```python
from build123d import *

# Parameters (mm, degrees)
SKETCH1_R           = 2
BOSS_EXTRUDE1_DEPTH = 2
BOSS_EXTRUDE2_START = -6
SKETCH2_R           = 3.5
SKETCH2_R_2         = 2
BOSS_EXTRUDE2_DEPTH = 4
BOSS_EXTRUDE3_START = 11
BOSS_EXTRUDE3_DEPTH = 11
BOSS_EXTRUDE4_START = -16
SKETCH5_R           = 2
BOSS_EXTRUDE4_DEPTH = 16


with BuildPart() as part:
    # Sketch1 → Boss-Extrude1 (new body)
    with BuildSketch(Plane.XY):
        with BuildLine():
            Line((-17.5, -10), (17.5, -10))
            ThreePointArc((17.5, -10), (23.235764364, -8.191520443), (26.896926208, -3.420201433))
            Line((26.896926208, -3.420201433), (40.065448474, 32.76001614))
            Line((40.065448474, 32.76001614), (-40.065448474, 32.76001614))
            Line((-40.065448474, 32.76001614), (-26.896926208, -3.420201433))
            ThreePointArc((-26.896926208, -3.420201433), (-23.235764364, -8.191520443), (-17.5, -10))
        make_face()
        with Locations((17.5, 0)):
            Circle(SKETCH1_R, mode=Mode.SUBTRACT)
        with Locations((-17.5, 0)):
            Circle(SKETCH1_R, mode=Mode.SUBTRACT)
        with BuildLine():
            Line((2.863480555, 21.190949642), (2.863480555, 7.014373782))
            ThreePointArc((2.863480555, 7.014373782), (0, 4.150893227), (-2.863480555, 7.014373782))
            Line((-2.863480555, 7.014373782), (-2.863480555, 21.190949642))
            ThreePointArc((-2.863480555, 21.190949642), (0, 24.054430197), (2.863480555, 21.190949642))
        make_face(mode=Mode.SUBTRACT)
    extrude(amount=BOSS_EXTRUDE1_DEPTH)

    # Sketch2 → Boss-Extrude2 (add)
    # profile 1 of 2: a face of its own
    with BuildSketch(Plane.XY.offset(2).offset(BOSS_EXTRUDE2_START)):
        with Locations((-17.5, 0)):
            Circle(SKETCH2_R)
        with Locations((-17.5, 0)):
            Circle(SKETCH2_R_2, mode=Mode.SUBTRACT)
    # profile 2 of 2: a face of its own
    with BuildSketch(Plane.XY.offset(2).offset(BOSS_EXTRUDE2_START)):
        with Locations((17.5, 0)):
            Circle(SKETCH2_R)
        with Locations((17.5, 0)):
            Circle(SKETCH2_R_2, mode=Mode.SUBTRACT)
    extrude(amount=BOSS_EXTRUDE2_DEPTH)

    # Sketch4 → Boss-Extrude3 (add)
    with BuildSketch(Plane(origin=(0, 0, 0), x_dir=(-1, 0, 0), z_dir=(0, 0, -1)).offset(BOSS_EXTRUDE3_START)):
        with BuildLine():
            Line((-26.896926208, -3.420201433), (-32.095820312, 10.863642724))
            Line((-32.095820312, 10.863642724), (-30.21643507, 11.547683011))
            Line((-30.21643507, 11.547683011), (-25.017540966, -2.736161147))
            ThreePointArc((-25.017540966, -2.736161147), (-22.088611491, -6.553216354), (-17.5, -8))
            Line((-17.5, -8), (-17.5, -10))
            ThreePointArc((-17.5, -10), (-23.235764364, -8.191520443), (-26.896926208, -3.420201433))
        make_face()
        with BuildLine():
            Line((32.095820312, 10.863642724), (26.896926208, -3.420201433))
            ThreePointArc((26.896926208, -3.420201433), (23.235764364, -8.191520443), (17.5, -10))
            Line((17.5, -10), (17.5, -8))
            ThreePointArc((17.5, -8), (22.088611491, -6.553216354), (25.017540966, -2.736161147))
            Line((25.017540966, -2.736161147), (30.21643507, 11.547683011))
            Line((30.21643507, 11.547683011), (32.095820312, 10.863642724))
        make_face()
    extrude(amount=-BOSS_EXTRUDE3_DEPTH)

    # Sketch5 → Boss-Extrude4 (add)
    with BuildSketch(Plane.XY.offset(2).offset(BOSS_EXTRUDE4_START)):
        with Locations((-17.5, 0)):
            Circle(SKETCH5_R)
        with Locations((17.5, 0)):
            Circle(SKETCH5_R)
    extrude(amount=BOSS_EXTRUDE4_DEPTH)


solid = part.part
```
The model under review builds one solid part; all positions refer to its coordinate system, in mm. A direction names the side the tool comes from. Round coordinates to 2 decimals unless told otherwise and drop trailing zeros. Order: outer loops, then holes, each group sorted by start corner. A loop starts at its lowest first (then second) coordinate and runs counter-clockwise, first axis right, second up. Notation, with made-up numbers: (-37.5, 13.25) -> (-28.5, 13.25) arc R12 cw to (-28.5, 34.25) -> close; hole circle Ø8 at (37, 45.25). An arc over 180 degrees is marked (long way). One line per item, written item: value. Start each with the question number.
Q1. Clearance check with flat-ended pins moving along their axes: pin 1 Ø0.6 at (y, z) = (-9.5, -7.5) entering from +X; pin 2 Ø7.5 at (x, y) = (26.5, 3.5) entering from -Z; pin 3 Ø8 at (x, z) = (-18.5, -6.5) entering from +Y; pin 4 Ø2 at (x, z) = (-11, -0.5) entering from +Y. State where each tip first meets the part, or that it passes through.
Q2. Wall thickness on line 1 (X direction, y = -0.5, z = -5.25); line 2 (Z direction, x = -27.5, y = 15); line 3 (X direction, y = 10, z = -7.25): over which ranges is each line inside the solid? List them lowest first.
Q3. Mouldability with a two-part tool opening along X and no side actions: class faces 5 (the face through (26, -1, -11)), 6 (the face through (20.84, 1.05, -2.03)), 7 (the face through (-23.31, -8.14, -4.59)) as released by +X, released by -X, zero draft, split by the parting line, or undercut.
Q4. Take a section at B-B (x = 0). Write out the cut boundary in (y, z).
Q5. Machinability: for faces 1 (the face through (-31.14, 11.21, -5.58)), 2 (the face through (31.17, 11.2, -5.58)), 3 (the face through (27.653, 4.506, -5.577)), 4 (the face through (-22.032, -6.592, -5.577)), which of the approach directions +Z, -Z, +X, -X, +Y, -Y give a long, thin tool a straight path to every point of the face, cutting with its end or side? Answer none if there is none.
Q6. Take a section at D-D (z = -13). Write out the cut boundary in (x, y).
Q7. Take a section at C-C (y = 13). Write out the cut boundary in (x, z), and give its area (3 significant figures).
Q8. Take a section at A-A (z = -5.75). Write out the cut boundary in (x, y).
Reported:
1. pin 1: stops at x = 21.42
1. pin 2: stops at z = -11
1. pin 3: stops at y = 3.5
1. pin 4: stops at y = 32.76
2. line 1: x = -27.96 to -25.83, -19.44 to -15.56, 15.56 to 19.44, 25.83 to 27.96
2. line 2: z = 0 to 2
2. line 3: x = -31.78 to -29.65, 29.65 to 31.78
3. face 5: zero draft
3. face 6: undercut
3. face 7: released by -X
4. outline: (-10, 0) -> (4.15, 0) -> (4.15, 2) -> (-10, 2) -> close; (24.05, 0) -> (32.76, 0) -> (32.76, 2) -> (24.05, 2) -> close
5. face 1: -Z, -X, +Y
5. face 2: -Z, +X, +Y
5. face 3: -Z, +Y
5. face 4: -Z
6. outline: circle Ø4 at (-17.5, 0); circle Ø4 at (17.5, 0)
7. outline: (-32.87, 0) -> (-2.86, 0) -> (-2.86, 2) -> (-32.87, 2) -> close; (2.86, 0) -> (32.87, 0) -> (32.87, 2) -> (2.86, 2) -> close
7. area: 120 mm2
8. outline: (-32.1, 10.86) -> (-26.9, -3.42) arc R10 ccw to (-17.5, -10) -> (-17.5, -8) arc R8 cw to (-25.02, -2.74) -> (-30.22, 11.55) -> close; circle Ø4 at (-17.5, 0); circle Ø4 at (17.5, 0); (17.5, -10) arc R10 ccw to (26.9, -3.42) -> (32.1, 10.86) -> (30.22, 11.55) -> (25.02, -2.74) arc R8 cw to (17.5, -8) -> close
